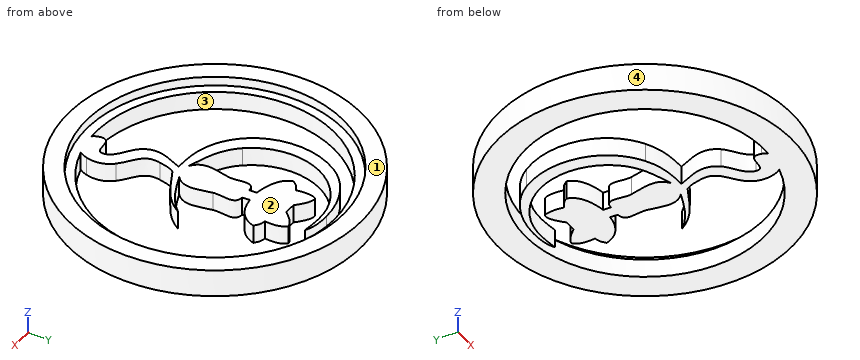
from build123d import *

# Parameters (mm, degrees)
PAD002_DEPTH  = 10
SKETCH_R      = 80
SKETCH_R_2    = 65
PAD_DEPTH     = 15
SKETCH001_R   = 70
SKETCH001_R_2 = 65
POCKET_DEPTH  = 5


with BuildPart() as design005:
    # Sketch004 → Pad002 (new body)
    with BuildSketch(Plane.XY):
        with BuildLine():
            add(Edge.make_bspline(
                [(2.857443, -18.112357), (-0.294933, -25.68391), (-5.159351, -33.231682), (0.976613, -40.898296)],
                knots=[0, 0, 0, 0, 1, 1, 1, 1], degree=3))
            add(Edge.make_bspline(
                [(0.976613, -40.898296), (4.258386, -44.998653), (11.444412, -47.145409), (12.433102, -52.81238)],
                knots=[0, 0, 0, 0, 1, 1, 1, 1], degree=3))
            add(Edge.make_bspline(
                [(12.433102, -52.81238), (13.672867, -59.918926), (0.142448, -52.599291), (2.448137, -61.936397)],
                knots=[0, 0, 0, 0, 1, 1, 1, 1], degree=3))
            add(Edge.make_bspline(
                [(2.448137, -61.936397), (4.168518, -68.902567), (12.92857, -67.682118), (16.678326, -63.34405)],
                knots=[0, 0, 0, 0, 1, 1, 1, 1], degree=3))
            add(Edge.make_bspline(
                [(16.678326, -63.34405), (17.9515, -61.871038), (18.73965, -60.086786), (19.252918, -58.224542)],
                knots=[0, 0, 0, 0, 1, 1, 1, 1], degree=3))
            add(Edge.make_bspline(
                [(19.252918, -58.224542), (20.62938, -53.230586), (19.684515, -48.0056), (16.087768, -44.18007)],
                knots=[0, 0, 0, 0, 1, 1, 1, 1], degree=3))
            add(Edge.make_bspline(
                [(16.087768, -44.18007), (10.550813, -38.291025), (2.704434, -36.922733), (4.725639, -27.026176)],
                knots=[0, 0, 0, 0, 1, 1, 1, 1], degree=3))
            add(Edge.make_bspline(
                [(4.725639, -27.026176), (5.25154, -24.448609), (5.856192, -20.447778), (7.733288, -18.49342)],
                knots=[0, 0, 0, 0, 1, 1, 1, 1], degree=3))
            add(Edge.make_bspline(
                [(7.733288, -18.49342), (17.735996, -13.502495), (26.919785, -9.769163), (32.570163, -0.28472)],
                knots=[0, 0, 0, 0, 1, 1, 1, 1], degree=3))
            add(Edge.make_bspline(
                [(32.570163, -0.28472), (26.066248, -7.456006), (18.281606, -10.206067), (9.542807, -13.655448)],
                knots=[0, 0, 0, 0, 1, 1, 1, 1], degree=3))
            add(Edge.make_bspline(
                [(9.542807, -13.655448), (16.000679, -8.525608), (13.223554, -1.474567), (11.713483, 6.058606)],
                knots=[0, 0, 0, 0, 1, 1, 1, 1], degree=3))
            add(Edge.make_bspline(
                [(11.713483, 6.058606), (10.782881, 10.701008), (14.934643, 19.337951), (7.8473, 19.546155)],
                knots=[0, 0, 0, 0, 1, 1, 1, 1], degree=3))
            add(Edge.make_bspline(
                [(7.8473, 19.546155), (7.456159, 23.596735)],
                knots=[0, 0, 1.449481, 1.449481], degree=1))
            add(Edge.make_bspline(
                [(7.456159, 23.596735), (15.213484, 24.396732), (21.533452, 27.885447), (23.656316, 35.370556)],
                knots=[0, 0, 0, 0, 1, 1, 1, 1], degree=3))
            add(Edge.make_bspline(
                [(23.656316, 35.370556), (21.738877, 36.918556), (20.996124, 37.847166), (17.967643, 38.191674)],
                knots=[0, 0, 0, 0, 1, 1, 1, 1], degree=3))
            add(Edge.make_bspline(
                [(17.967643, 38.191674), (18.163326, 41.416764), (18.577573, 46.391209), (15.485334, 49.484093)],
                knots=[0, 0, 0, 0, 1, 1, 1, 1], degree=3))
            add(Edge.make_bspline(
                [(15.485334, 49.484093), (11.619572, 49.321819), (6.684433, 42.943063), (6.684433, 42.943063)],
                knots=[0, 0, 0, 0, 1, 1, 1, 1], degree=3))
            add(Edge.make_bspline(
                [(6.684433, 42.943063), (0.389929, 42.975068)],
                knots=[0, 0, 2.242059, 2.242059], degree=1))
            add(Edge.make_bspline(
                [(0.389929, 42.975068), (0.389929, 42.975068), (-5.357645, 49.546785), (-9.404462, 48.888341)],
                knots=[0, 0, 0, 0, 1, 1, 1, 1], degree=3))
            add(Edge.make_bspline(
                [(-9.404462, 48.888341), (-11.478785, 46.3327), (-10.479708, 39.424645), (-10.082306, 37.964604)],
                knots=[0, 0, 0, 0, 1, 1, 1, 1], degree=3))
            add(Edge.make_bspline(
                [(-10.082306, 37.964604), (-11.769249, 37.110168), (-13.705696, 36.218281), (-15.379613, 33.344635)],
                knots=[0, 0, 0, 0, 1, 1, 1, 1], degree=3))
            add(Edge.make_bspline(
                [(-15.379613, 33.344635), (-14.000933, 27.134412), (-5.854881, 24.350493), (1.003565, 23.442238)],
                knots=[0, 0, 0, 0, 1, 1, 1, 1], degree=3))
            add(Edge.make_bspline(
                [(1.003565, 23.442238), (1.210197, 19.360017)],
                knots=[0, 0, 1.455902, 1.455902], degree=1))
            add(Edge.make_bspline(
                [(1.210197, 19.360017), (-6.253659, 19.181741), (-1.456845, 10.612599), (-2.443795, 5.974016)],
                knots=[0, 0, 0, 0, 1, 1, 1, 1], degree=3))
            add(Edge.make_bspline(
                [(-2.443795, 5.974016), (-4.454668, -3.477046), (-6.614086, -9.8608), (-0.113933, -14.398285)],
                knots=[0, 0, 0, 0, 1, 1, 1, 1], degree=3))
            add(Edge.make_bspline(
                [(-0.113933, -14.398285), (-9.732856, -11.135827), (-18.226675, -8.719438), (-24.872819, -0.284748)],
                knots=[0, 0, 0, 0, 1, 1, 1, 1], degree=3))
            add(Edge.make_bspline(
                [(-24.872819, -0.284748), (-38.713975, 17.282017), (-33.70723, 44.153601), (-13.484661, 54.695238)],
                knots=[0, 0, 0, 0, 1, 1, 1, 1], degree=3))
            add(Edge.make_bspline(
                [(-13.484661, 54.695238), (-4.122569, 59.575547), (3.993106, 58.947368), (13.999604, 57.655075)],
                knots=[0, 0, 0, 0, 1, 1, 1, 1], degree=3))
            add(Edge.make_bspline(
                [(13.999604, 57.655075), (9.88215, 60.2423), (4.647534, 60.620555), (-0.113933, 60.626339)],
                knots=[0, 0, 0, 0, 1, 1, 1, 1], degree=3))
            add(Edge.make_bspline(
                [(-0.113933, 60.626339), (-12.760213, 60.643184), (-26.055459, 55.212155), (-33.133851, 44.284347)],
                knots=[0, 0, 0, 0, 1, 1, 1, 1], degree=3))
            add(Edge.make_bspline(
                [(-33.133851, 44.284347), (-45.363462, 25.403755), (-41.088394, -1.481951), (-20.912857, -13.102089)],
                knots=[0, 0, 0, 0, 1, 1, 1, 1], degree=3))
            add(Edge.make_bspline(
                [(-20.912857, -13.102089), (-13.292123, -17.490636), (-5.714956, -18.112386), (2.857331, -18.112386)],
                knots=[0, 0, 0, 0, 1, 1, 1, 1], degree=3))
            add(Edge.make_bspline(
                [(2.857331, -18.112386), (2.857443, -18.112357)],
                knots=[0, 0, 4.1e-05, 4.1e-05], degree=1))
        make_face()
    extrude(amount=PAD002_DEPTH)


with BuildPart() as half_lamp_with_design:
    # Sketch → Pad (new body)
    with BuildSketch(Plane.XY):
        Circle(SKETCH_R)
        Circle(SKETCH_R_2, mode=Mode.SUBTRACT)
    extrude(amount=PAD_DEPTH)

    # Sketch001 (on Face4 of Pad) → Pocket (cut)
    with BuildSketch(Plane.XY.offset(15)):
        Circle(SKETCH001_R)
        Circle(SKETCH001_R_2, mode=Mode.SUBTRACT)
    extrude(amount=-POCKET_DEPTH, mode=Mode.SUBTRACT)

    # Boolean: union design005
    add(design005.part)


solid = half_lamp_with_design.part
For this review, take the finished solid that the model builds, in its own axes (mm). Face numbers are marked on the shaded views. Round coordinates to 2 decimals unless told otherwise and drop trailing zeros. Write each loop counter-clockwise with the first axis right and the second up, starting at its lowest first coordinate (ties: lowest second). Pieces come first, ordered by that corner, then holes. Notation, with made-up numbers: (64.5, 50.5) - (97.5, 50.5) arc R28 ccw to (97.5, 76.5) - close; hole circle Ø7 at (24, 22.25). An arc over 180 degrees is marked (long way). Write item = value, one per line. Start each with the question number.
1. Consider section C-C on x = -51. State the section outline as (y, z) points.
2. Consider section B-B on y = 41. Give the number of separate pieces and of enclosed holes in the cut face, plus the area to 3 significant figures.
3. Consider section A-A on x = 53.5. State the section outline as (y, z) points.
4. For pin 1 Ø8 at (y, z) = (11.5, 7) entering from -X; pin 2 Ø1.5 at (y, z) = (-22.5, 9.5) entering from +X; pin 3 Ø2 at (y, z) = (-13.5, 11) entering from -X, all flat-tipped, find the tip position at first contact; note any pin that passes through.
5. Draft analysis for pull direction X (two halves, no side actions). For the marked faces 1, 2, 3 and 4, state which applies: released by +X, released by -X, zero draft, split by the parting line, or undercut.
6. Wall thickness on L1, parallel to Y at x = 0, z = 11.1; L2, parallel to X at y = -5, z = 4; L3, parallel to Y at x = 0, z = 7.5: over which ranges is each line inside the solid? List them lowest first.
Evaluation:
q1.outline = (-61.64, 0) - (-40.3, 0) - (-40.3, 10) - (-47.95, 10) - (-47.95, 15) - (-61.64, 15) - close; (40.3, 0) - (61.64, 0) - (61.64, 15) - (47.95, 15) - (47.95, 10) - (40.3, 10) - close
q2.separate_pieces = 4
q2.enclosed_holes = 0
q2.area = 844 mm2
q3.outline = (-59.48, 0) - (-36.92, 0) - (-36.92, 10) - (-45.14, 10) - (-45.14, 15) - (-59.48, 15) - close; (36.92, 0) - (59.48, 0) - (59.48, 15) - (45.14, 15) - (45.14, 10) - (36.92, 10) - close
q4.pin_1 = -79.65
q4.pin_2 = 76.99
q4.pin_3 = -79.02
q5.face_1 = zero draft
q5.face_2 = undercut
q5.face_3 = undercut
q5.face_4 = split by the parting line
q6.L1 = -80 to -70, 70 to 80
q6.L2 = -79.84 to -64.81, -30.67 to -20.29, -4.44 to 13.62, 27.34 to 29.09, 64.81 to 79.84
q6.L3 = -80 to -65, -39.54 to -24.68, -18.08 to 19.24, 23.59 to 43.4, 58.49 to 60.63, 65 to 80
